Model file for the job. Use its own axes, mm. Face numbers are marked on the shaded views. A direction names the side the tool comes from. Coordinates: 2 decimals unless noted, no trailing zeros. Order: outer loops, then holes, each group sorted by start corner. A loop starts at its lowest first (then second) coordinate and runs counter-clockwise, first axis right, second up. Notation, with made-up numbers: (82, 42.25) -> (120, 42.25) arc R35 ccw to (120, 75.25) -> close; hole circle Ø9 at (17, 7.25). An arc over 180 degrees is marked (long way). Write item = value, one per line. Start each with the question number.
Q1. Flat gauge pins, fed straight in: pin 1 (2 mm diameter, centred on x = 122.2, y = 193.68, fed in from -Z); pin 2 (2 mm diameter, centred on x = 168, z = 182.5, fed in from -Y). Where does each tip first touch, or does it go through?
Q2. Wall check: line 1 (Y direction, x = 118, z = 189.5); line 2 (X direction, y = 12.5, z = 51). Give the ranges that are in metal, low to high. Write a range as from..to.
Q3. 3-axis set-ups, long thin cutter, end or side, ignore diameter. For the marked faces 1 and 2: which of +Z, -Z, +X, -X, +Y, -Y reach the whole face in a straight line?
Q4. Cut at B-B, the plane y = 220.5. List the corners of the cut face in (x, z), plus the area to 3 significant figures.
Q5. Cut at D-D, the plane x = 128.5. List the corners of the cut face in (y, z) (3 decimals).
Q6. Mould opens along Y. For the marked faces 3, 4 and 5 say: +Y half, -Y half, draft (parallel to the pull), parting line (faces both ways), or undercut.
Q7. Cut at C-C, the plane z = 127.5. List the corners of the cut face in (x, y), plus the area to 3 significant figures.
Q8. Cut at A-A, the plane x = 100.33. List the corners of the cut face in (y, z) (3 decimals), plus the area to 3 significant figures.
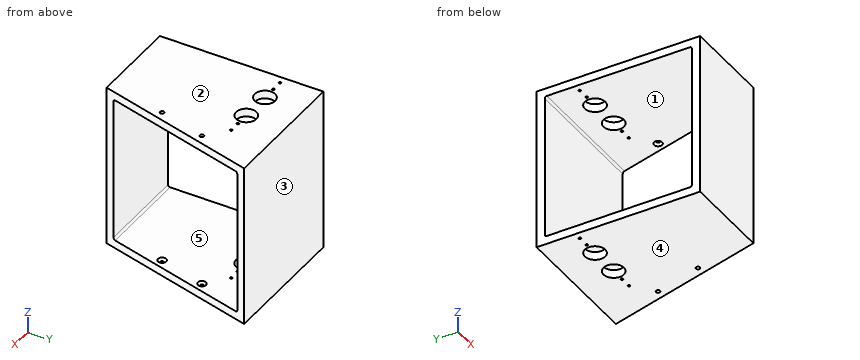
Autodesk Inventor part; units mm, degrees
ref_plane "YZ Plane" through (0, 0, 0) normal (1, 0, 0) x (0, 1, 0)
ref_plane "XZ Plane" through (0, 0, 0) normal (0, 1, 0) x (-1, 0, 0)
ref_plane "XY Plane" through (0, 0, 0) normal (0, 0, 1) x (1, 0, 0)
sketch "Sketch1" plane through (0, 0, 0) normal (0, 0, 1) x (1, 0, 0)
  line L0 (0, 0) -> (0, 254)
  line L1 (0, 254) -> (207.7591, 254)
  line L2 (207.7591, 254) -> (139.7, 0)
  line L3 (139.7, 0) -> (0, 0)
  dimension "d0" = 254
  dimension "d2" = 139.7
  dimension "d24" = 75
extrude "Extrusion1" add sketch "Sketch1" along normal blind 254
sketch "Sketch2" plane through (0, 0, 0) normal (-1, 0, 0) x (0, 0, 1)
  line L0 (254, 0) -> (254, 254)
  line L1 (0, 254) -> (254, 254)
  line L2 (0, 0) -> (0, 254)
  line L3 (0, 0) -> (254, 0)
  line L4 (241.3, 241.3) -> (241.3, 12.7)
  line L5 (241.3, 12.7) -> (12.7, 12.7)
  line L6 (12.7, 12.7) -> (12.7, 241.3)
  line L7 (12.7, 241.3) -> (241.3, 241.3)
  dimension "d5" = 12.7
extrude "Extrusion2" cut sketch "Sketch2" against normal blind 209.55 contours L4 L5 L6 L7
sketch "Sketch6" plane through (0, 12.7, 241.3) normal (0, 0, -1) x (-1, 0, 0)
  line L0 (-143.103, 0) -> (-204.3561, 228.6)
  line L1 (0, 241.3) -> (-207.7591, 241.3)
  line L2 (-207.7591, 241.3) -> (-191.6487, 245.6168)
  point P0 (0, -12.7)
  point P1 (-139.7, -12.7)
  point P2 (-171.2502, 154.116)
  point P3 (-151.5282, 80.5124)
  point P4 (-203.2, 224.2852)
  dimension "d73" = 93.6625
  dimension "d74" = 169.8625
  dimension "d75" = 12.7
  dimension "d76" = 12.7
sketch "Sketch7" plane through (0, 12.7, 12.7) normal (0, 0, 1) x (1, 0, 0)
  point P0 (0, -12.7)
  point P1 (171.2502, 154.116)
  point P2 (151.5282, 80.5124)
hole "Hole1" at (51.435, 193.675, 254) direction (0, 0, -1) diameter 31.75 end through all
hole "Hole2" at (171.2502, 166.816, 12.7) direction (0, 0, -1) diameter 6.35 depth 25.4 tip angle 118 countersink diameter 12.7 countersink angle 82
hole "Hole3" at (151.5282, 93.2124, 12.7) direction (0, 0, -1) diameter 6.35 depth 25.4 tip angle 118 countersink diameter 12.7 countersink angle 82
hole "Hole4" at (171.2502, 166.816, 241.3) direction (0, 0, 1) diameter 6.35 depth 25.4 tip angle 118 countersink diameter 12.7 countersink angle 82
hole "Hole5" at (151.5282, 93.2124, 241.3) direction (0, 0, 1) diameter 6.35 depth 25.4 tip angle 118 countersink diameter 12.7 countersink angle 82
fillet "Fillet1" radius 3.175 4 edges at (102.1781, 241.3, 12.7) (102.1781, 241.3, 241.3) (71.5515, 12.7, 241.3) (71.5515, 12.7, 12.7)
pattern_linear "Rectangular Pattern2" count 2 spacing 48.895 along (1, 0, 0) of "Hole1"
hole "Hole6" at (29.4894, 193.675, 254) direction (0, 0, -1) diameter 3.683 end through all
pattern_linear "Rectangular Pattern3" count 2 spacing 17.78 along (-1, 0, 0) of "Hole6"
pattern_linear "Rectangular Pattern4" count 2 spacing 110.49 along (1, 0, 0) of "Hole6", "Rectangular Pattern3"
properties part number "GE-12059"
Here are the results:
q1.pin_1 = through
q1.pin_2 = 241.3
q2.line_1 = 0..12.7, 241.3..254
q2.line_2 = 0..143.05
q3.face_1 = +X, -X
q3.face_2 = +Z, +X, -X, +Y, -Y
q4.outline = (0, 0) -> (198.78, 0) -> (198.78, 12.7) -> (0, 12.7) -> close; (0, 241.3) -> (198.78, 241.3) -> (198.78, 254) -> (0, 254) -> close
q4.area = 5,050 mm²
q5.outline = (0, 0) -> (254, 0) -> (254, 254) -> (0, 254) -> close; hole (12.7, 15.875) arc R3.175 ccw to (15.875, 12.7) -> (238.125, 12.7) arc R3.175 ccw to (241.3, 15.875) -> (241.3, 238.125) arc R3.175 ccw to (238.125, 241.3) -> (15.875, 241.3) arc R3.175 ccw to (12.7, 238.125) -> close
q6.face_3 = +Y half
q6.face_4 = draft
q6.face_5 = undercut
q7.outline = (0, 0) -> (139.7, 0) -> (143.1, 12.7) -> (0, 12.7) -> close; (0, 241.3) -> (204.36, 241.3) -> (207.76, 254) -> (0, 254) -> close
q7.area = 4,410 mm²
q8.outline = (0, 0) -> (177.8, 0) -> (177.8, 12.7) -> (15.875, 12.7) arc R3.175 cw to (12.7, 15.875) -> (12.7, 238.125) arc R3.175 cw to (15.875, 241.3) -> (177.8, 241.3) -> (177.8, 254) -> (0, 254) -> close; (209.55, 0) -> (254, 0) -> (254, 254) -> (209.55, 254) -> (209.55, 241.3) -> (238.125, 241.3) arc R3.175 cw to (241.3, 238.125) -> (241.3, 15.875) arc R3.175 cw to (238.125, 12.7) -> (209.55, 12.7) -> close
q8.area = 11,500 mm²
